from build123d import *


with BuildPart() as part:
    # Sketch1 → Revolve7 (revolve)
    with BuildSketch(Plane(origin=(0, 0, 0), x_dir=(1, 0, 0), z_dir=(0, 1, 0))):
        with BuildLine():
            Line((0, 66), (0, 110))
            ThreePointArc((0, 110), (38.823317736, 107.489546564), (77, 100))
            Line((77, 100), (77, 93))
            Line((77, 93), (70, 93))
            Line((70, 93), (70, 84))
            Line((70, 84), (77, 84))
            Line((77, 84), (77, 75))
            Line((77, 75), (70, 75))
            Line((70, 75), (70, 66))
            Line((70, 66), (77, 66))
            Line((77, 66), (77, 0))
            Line((77, 0), (67, 0))
            Line((67, 0), (67, 16))
            Line((67, 16), (52.5, 16))
            Line((52.5, 16), (52.5, 66))
            Line((52.5, 66), (0, 66))
        make_face()
    revolve(axis=Axis((0, 0, 14.193325573), (0, 0, -1)))


solid = part.part
Model file for the job. Use its own axes, mm. A direction names the side the tool comes from. Give positions to 0.01 mm unless a question says otherwise; leave off trailing zeros. Order: outer loops, then holes, each group sorted by start corner. A loop starts at its lowest first (then second) coordinate and runs counter-clockwise, first axis right, second up. Notation, with made-up numbers: (26, -35.5) - (84, -35.5) arc R5 ccw to (84, -27.5) - close; hole circle Ø11 at (76, 32). An arc over 180 degrees is marked (long way). Write item = value, one per line. Start each with the question number.
1. Two-plate mould, pull along X, no slides. Class faces 1 (the flat face through (17.5, 68.1, -66)), 2 (the cylindrical face through (-14.524, 65.407, -8.112)), 3 (the cylindrical face through (-61.105, 46.853, -96.451)): pulls with the +X half, pulls with the -X half, needs draft (parallel to the pull), parting line crosses it, or undercut.
2. Which spindle directions (+Z, -Z, +X, -X, +Y, -Y) get a long thin tool onto all of the face, cutting with end or side? Do faces 4 (the cylindrical face through (-61.105, 46.853, -79.437)), 5 (the cylindrical face through (-55.55, 42.594, -70.437)), 6 (the cylindrical face through (50.076, -15.77, -41.35)). Say none if no direction does.
3. Probe line 1 along X through (y, z) = (0, -10); line 2 along Z through (x, y) = (56, 50). List the from-to ranges inside material, lowest first.
4. Drop flat-ended pins along their axis: P1, Ø4, axis at x = -31, z = -17.5, coming from the -Y side; P2, Ø2, axis at x = -21.5, y = -37.5, coming from the +Z side; P3, Ø3, axis at x = -32, y = 33.5, coming from the -Z side. Give the stop position or say it passes through.
5. Cut at D-D, the plane z = -9. List the corners of the cut face in (x, y).
6. Cut at A-A, the plane x = 0. List the corners of the cut face in (y, z), and give its area (3 significant figures).
7. Cut at C-C, the plane z = -79. List the corners of the cut face in (x, y).
Taken from the geometry:
q1.face_1 = needs draft
q1.face_2 = undercut
q1.face_3 = parting line crosses it
q2.face_4 = +Z, -Z
q2.face_5 = none
q2.face_6 = +Z
q3.line_1 = -77 to -67, 67 to 77
q3.line_2 = -100.5 to -93, -84 to -75, -66 to 0
q4.P1 = -71.33
q4.P2 = -66
q4.P3 = -106.65
q5.outline = circle Ø154 at (0, 0); hole circle Ø134 at (0, 0)
q6.outline = (-77, -100) arc R301.45 ccw to (77, -100) - (77, -93) - (70, -93) - (70, -84) - (77, -84) - (77, -75) - (70, -75) - (70, -66) - (77, -66) - (77, 0) - (67, 0) - (67, -16) - (52.5, -16) - (52.5, -66) - (-52.5, -66) - (-52.5, -16) - (-67, -16) - (-67, 0) - (-77, 0) - (-77, -66) - (-70, -66) - (-70, -75) - (-77, -75) - (-77, -84) - (-70, -84) - (-70, -93) - (-77, -93) - close
q6.area = 8,780 mm²
q7.outline = circle Ø154 at (0, 0)
